from build123d import *

# Parameters (mm, degrees)
BOX001_W        = 3
BOX001_H        = 4
BOX001_DEPTH    = 5
CHAMFER_SIZE    = 2
BOX002_W        = 2
BOX002_H        = 8
BOX002_DEPTH    = 1
CHAMFER001_SIZE = 1.8
SKETCH004_W     = 1
SKETCH004_H     = 14
PAD004_DEPTH    = 1
SKETCH005_W     = 28
SKETCH005_H     = 1
PAD005_DEPTH    = 1
SKETCH006_W     = 1
SKETCH006_H     = 14
PAD006_DEPTH    = 1
SKETCH003_W     = 28
SKETCH003_H     = 1
PAD003_DEPTH    = 1
BOX_W           = 28
BOX_H           = 14
BOX_DEPTH       = 0.125


with BuildPart() as chamfer_body:
    # Box001 → Box001 (new body)
    with BuildSketch(Plane(origin=(-1, 5, 0.125), x_dir=(1, 0, 0), z_dir=(0, 0, 1))):
        with Locations((1.5, 2)):
            Rectangle(BOX001_W, BOX001_H)
    extrude(amount=BOX001_DEPTH)

    # Chamfer
    chamfer_edges = [chamfer_body.edges().sort_by_distance(p)[0] for p in [
        (-1, 7, 0.125),
    ]]
    chamfer(chamfer_edges, length=CHAMFER_SIZE)


with BuildPart() as chamfer001:
    # Box002 → Box002 (new body)
    with BuildSketch(Plane(origin=(-2, 3, 0), x_dir=(1, 0, 0), z_dir=(0, 0, 1))):
        with Locations((1, 4)):
            Rectangle(BOX002_W, BOX002_H)
    extrude(amount=BOX002_DEPTH)

    # Chamfer001
    chamfer001_edges = [chamfer001.edges().sort_by_distance(p)[0] for p in [
        (-2, 3, 0.5),
        (-2, 11, 0.5),
    ]]
    chamfer(chamfer001_edges, length=CHAMFER001_SIZE)


with BuildPart() as pad004:
    # Sketch004 → Pad004 (new body)
    with BuildSketch(Plane.XY.offset(0.125)):
        with Locations((0.5, 7)):
            Rectangle(SKETCH004_W, SKETCH004_H)
    extrude(amount=PAD004_DEPTH)


with BuildPart() as pad005:
    # Sketch005 → Pad005 (new body)
    with BuildSketch(Plane.XY.offset(0.125)):
        with Locations((14, 0.5)):
            Rectangle(SKETCH005_W, SKETCH005_H)
    extrude(amount=PAD005_DEPTH)


with BuildPart() as pad006:
    # Sketch006 → Pad006 (new body)
    with BuildSketch(Plane.XY.offset(0.125)):
        with Locations((27.5, 7)):
            Rectangle(SKETCH006_W, SKETCH006_H)
    extrude(amount=PAD006_DEPTH)


with BuildPart() as walls:
    # Sketch003 → Pad003 (new body)
    with BuildSketch(Plane.XY.offset(0.125)):
        with Locations((14, 13.5)):
            Rectangle(SKETCH003_W, SKETCH003_H)
    extrude(amount=PAD003_DEPTH)

    # Fusion001: union Pad004, Pad005, Pad006
    add(pad004.part)
    add(pad005.part)
    add(pad006.part)

    # Fusion: union Chamfer001
    add(chamfer001.part)

    # Cut: cut Chamfer body
    add(chamfer_body.part, mode=Mode.SUBTRACT)


with BuildPart() as base_and_walls_do_not_edit:
    # Box → Box (new body)
    with BuildSketch(Plane.XY):
        with Locations((14, 7)):
            Rectangle(BOX_W, BOX_H)
    extrude(amount=BOX_DEPTH)

    # Fusion024: union Walls
    add(walls.part)


solid = base_and_walls_do_not_edit.part
Work out the finished part from the listing and answer in its coordinate system (mm). A direction names the side the tool comes from. Coordinates: 2 decimals unless noted, no trailing zeros. Write each loop counter-clockwise with the first axis right and the second up, starting at its lowest first coordinate (ties: lowest second). Pieces come first, ordered by that corner, then holes. Notation, with made-up numbers: M 34.5,-40 L 71.5,-40 A18 cw 71.5,-29 Z; hole C 44.25,12.5 d8. An arc over 180 degrees is marked long. Use one line per item in the form item = value. Start each with the question number.
1. The part is cut by section B-B (x = 15.25). Give the vertices of the cut face in (y, z) (3 decimals).
2. Straight lines are drawn through the part: probe 1 along X at (y, z) = (2.5, 0.6); probe 2 along Y at (x, z) = (2.75, 0.55); probe 3 along X at (y, z) = (9.5, 0.55). For each, find the intervals that lie inside material, in ascending order. Write a range as from..to.
3. The mould has two halves that part along X. Classify faces 1 (the face through (-1, 7, 1)), 2 (the face through (-1.1, 10.1, 0.5)), 3 (the face through (13.8, 1, 0.6)): released by +X, released by -X, zero draft, split by the parting line, or undercut.
4. The part is cut by section D-D (y = 1.5). Give the vertices of the cut face in (x, z) (3 decimals), plus the area to 3 significant figures.
5. The part is cut by section A-A (y = 10). Give the vertices of the cut face in (x, z) (3 decimals).
6. Each of these flat-tipped pins is pushed along its axis until it touches: P1, Ø8, axis at x = 22.5, y = 6.5, coming from the +Z side (3 decimals); P2, Ø1, axis at x = -1, y = 6.5, coming from the +Z side. Where does it stop, or does it pass through?
7. The part is cut by section C-C (z = 0.35). Give the vertices of the cut face in (x, y) (3 decimals).
8. A tool of negligible diameter and unlimited length cuts with its end or side. For faces 4 (the face through (28, 6.9, 0.6)), 5 (the face through (1, 11, 0.6)), from which of +Z, -Z, +X, -X, +Y, -Y can it reach the whole face along a straight path? Write none if from no direction.
Evaluation:
q1.outline = M 0,0 L 14,0 L 14,1.125 L 13,1.125 L 13,0.125 L 1,0.125 L 1,1.125 L 0,1.125 Z
q2.probe_1 = 0..1, 27..28
q2.probe_2 = 0..1, 13..14
q2.probe_3 = -1.7..1, 27..28
q3.face_1 = zero draft
q3.face_2 = released by -X
q3.face_3 = undercut
q4.outline = M 0,0 L 28,0 L 28,1.125 L 27,1.125 L 27,0.125 L 1,0.125 L 1,1.125 L 0,1.125 Z
q4.area = 5.50 mm^2
q5.outline = M -1.2,0 L 28,0 L 28,1.125 L 27,1.125 L 27,0.125 L 1,0.125 L 1,1.125 L 0,1.125 L 0,1 L -1.2,1 Z
q6.P1 = 0.125
q6.P2 = 1
q7.outline = M -2,4.8 L -0.2,3 L 0,3 L 0,0 L 28,0 L 28,14 L 0,14 L 0,11 L -0.2,11 L -2,9.2 Z; hole M 0.775,5 L 1,5 L 1,1 L 27,1 L 27,13 L 1,13 L 1,9 L 0.775,9 Z
q8.face_4 = +Z, -Z, +X, +Y, -Y
q8.face_5 = +Z
